Autodesk Inventor part; units mm, degrees
ref_plane "YZ Plane" through (0, 0, 0) normal (1, 0, 0) x (0, 1, 0)
ref_plane "XZ Plane" through (0, 0, 0) normal (0, 1, 0) x (-1, 0, 0)
ref_plane "XY Plane" through (0, 0, 0) normal (0, 0, 1) x (1, 0, 0)
sketch "Sketch2" plane through (0, 0, 0) normal (0, 0, 1) x (1, 0, 0)
  line L0 (11.5, 0) -> (35.5, 0)
  line L1 (35.5, 0) -> (35.5, 4)
  line L2 (35.5, 4) -> (21.5, 4)
  line L3 (21.5, 4) -> (16, 14)
  line L4 (16, 14) -> (13, 14)
  line L5 (13, 14) -> (13, 6)
  line L6 (13, 6) -> (11.5, 6)
  line L7 (11.5, 6) -> (11.5, 0)
  line L8 (0, -2.8) -> (0, 16.8)
  point P0 (0, 0)
  dimension "d0" = 13
  dimension "d1" = 1.5
  dimension "d2" = 3
  dimension "d3" = 24
  dimension "d4" = 6
  dimension "d5" = 8
  dimension "d6" = 0
  dimension "d7" = 4
  dimension "d8" = 14
revolve "Revolution1" add sketch "Sketch2" angle 360 about axis through (0, -10, 0) along (0, 1, 0)
properties part number "base reaction wheel" material "ABS Plastic"
CAD build for the part. Positions are in the model's coordinates, mm. A direction names the side the tool comes from. Round coordinates to 2 decimals unless told otherwise and drop trailing zeros. Loops run counter-clockwise (first coordinate to the right, second up) from the corner with the lowest first, then second, coordinate; pieces in that order, holes last.
(1) Cut at C-C (y = 3). Give the cut face in (x, z), plus the area to 3 significant figures.
(2) Cut at A-A (x = 0). Give the cut face in (y, z).
(3) Cut at D-D (z = -25). Give the cut face in (x, y), plus the area to 3 significant figures.
(4) Drop flat-ended pins along their axis: pin 1 (8 mm diameter, centred on x = -5.5, z = 3.5, fed in from +Y); pin 2 (4 mm diameter, centred on x = -11, y = 3.5, fed in from -Z); pin 3 (1.5 mm diameter, centred on x = -9, y = 12, fed in from +Z); pin 4 (1 mm diameter, centred on x = 17.5, y = 2, fed in from -Z). Give the stop position or say it passes through.
(5) Cut at B-B (z = 0). Give the cut face in (x, y).
(6) Two-plate mould, pull along Z, no slides. Class faces 3 (the flat face through (0, 4, 23)), 4 (the conical face through (-3.54, 13.37, -15.96)), 5 (the flat face through (5, 6, 11)): +Z half, -Z half, draft (parallel to the pull), parting line (faces both ways), or undercut.
(7) Wall check: line 1 along X through (y, z) = (3, 0); line 2 along Y through (x, z) = (7.5, -31.5); line 3 along Y through (x, z) = (8, 9.5). Give the ranges that are in metal, low to high.
(8) Which spindle directions (+Z, -Z, +X, -X, +Y, -Y) get a long thin tool onto all of the face, cutting with end or side? Do faces 1 (the flat face through (-1.3, 14, -13.1)), 2 (the cylindrical face through (-10.316, 9.944, -7.91)). Say none if no direction does.
Findings below:
1. outline: circle Ø71 at (0, 0); hole circle Ø23 at (0, 0)
1. area: 3,540 mm2
2. outline: (0, -35.5) - (4, -35.5) - (4, -21.5) - (14, -16) - (14, -13) - (6, -13) - (6, -11.5) - (0, -11.5) - close; (0, 11.5) - (6, 11.5) - (6, 13) - (14, 13) - (14, 16) - (4, 21.5) - (4, 35.5) - (0, 35.5) - close
3. outline: (-25.2, 0) - (25.2, 0) - (25.2, 4) - (-25.2, 4) - close
3. area: 202 mm2
4. pin 1: passes through
4. pin 2: stops at z = -34.34
4. pin 3: stops at z = 15.19
4. pin 4: stops at z = -31.16
5. outline: (-35.5, 0) - (-11.5, 0) - (-11.5, 6) - (-13, 6) - (-13, 14) - (-16, 14) - (-21.5, 4) - (-35.5, 4) - close; (11.5, 0) - (35.5, 0) - (35.5, 4) - (21.5, 4) - (16, 14) - (13, 14) - (13, 6) - (11.5, 6) - close
6. face 3: draft
6. face 4: parting line
6. face 5: undercut
7. line 1: x = -35.5 to -11.5, 11.5 to 35.5
7. line 2: y = 0 to 4
7. line 3: y = 0 to 6
8. face 1: +Z, -Z, +X, -X, +Y
8. face 2: +Y
